Build history of the part. All positions in model axes, mm. Face numbers are marked on the shaded views. Coordinates: 2 decimals unless noted, no trailing zeros. Loops run counter-clockwise (first coordinate to the right, second up) from the corner with the lowest first, then second, coordinate; pieces in that order, holes last. Notation, with made-up numbers: M 25,-29.5 L 61,-29.5 A20 cw 61,-16.5 Z; hole C -11.5,35 d5. An arc over 180 degrees is marked long. Write each question's results on one line, items separated by ' | '. Start each with the question number.
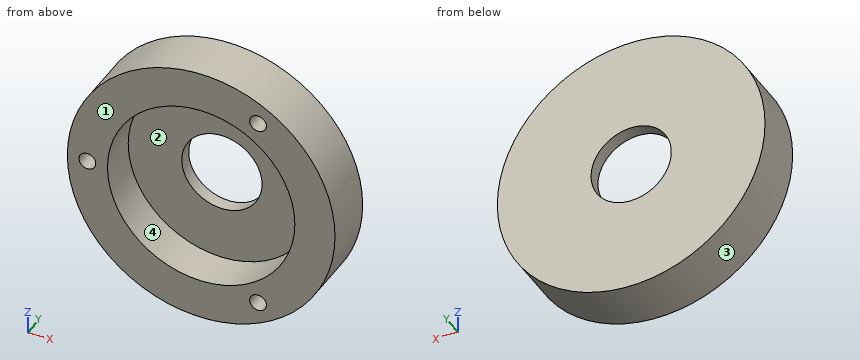
from build123d import *

# Parameters (mm, degrees)
SKETCH1_R                 = 20
BOSS_EXTRUDE1_DEPTH       = 8
SKETCH2_R                 = 14
CUT_EXTRUDE1_DEPTH        = 6
CUT_EXTRUDE4_REACH        = 10
SKETCH3_R                 = 6
M3X0_5_TAPPED_HOLE1_D     = 2.5
M3X0_5_TAPPED_HOLE1_DEPTH = 4
M3X0_5_TAPPED_HOLE1_TIP   = 0.751075774


with BuildPart() as part:
    # Sketch1 → Boss-Extrude1 (new body)
    with BuildSketch(Plane(origin=(0, 3, 0), x_dir=(1, 0, 0), z_dir=(0, 1, 0))):
        with Locations((-34.143225555, -5.12970783)):
            Circle(SKETCH1_R)
    extrude(amount=BOSS_EXTRUDE1_DEPTH)

    # Sketch2 → Cut-Extrude1 (cut)
    with BuildSketch(Plane.XZ.offset(-3)):
        with Locations((-34.143225555, 5.12970783)):
            Circle(SKETCH2_R)
    extrude(amount=-CUT_EXTRUDE1_DEPTH, mode=Mode.SUBTRACT)

    # Sketch3 → Cut-Extrude4 (cut, up to next)
    with BuildSketch(Plane(origin=(0, 11, 0), x_dir=(1, 0, 0), z_dir=(0, 1, 0)), mode=Mode.PRIVATE) as cut_extrude4_sk1:
        with Locations((-34.143225555, -5.12970783)):
            Circle(SKETCH3_R)
    cut_extrude4_tool1 = extrude(cut_extrude4_sk1.sketch, amount=-CUT_EXTRUDE4_REACH, mode=Mode.PRIVATE) & part.part
    add(cut_extrude4_tool1.solids().sort_by_distance((-34.143226, 11, 5.129708))[0], mode=Mode.SUBTRACT)

    # M3x0.5 Tapped Hole1
    with Locations(Plane.XZ.offset(-3)):
        with Locations((-25.643225555, 19.852139695), (-51.143225555, 5.12970783), (-25.643225555, -9.592724034)):
            Hole(M3X0_5_TAPPED_HOLE1_D / 2, depth=M3X0_5_TAPPED_HOLE1_DEPTH)
            with Locations((0, 0, -(M3X0_5_TAPPED_HOLE1_DEPTH + M3X0_5_TAPPED_HOLE1_TIP / 2))):  # 118° drill point
                Cone(0, M3X0_5_TAPPED_HOLE1_D / 2, M3X0_5_TAPPED_HOLE1_TIP, mode=Mode.SUBTRACT)


solid = part.part
1. Mould opens along Z. For the marked faces 1, 2, 3 and 4 say: +Z half, -Z half, draft (parallel to the pull), parting line (faces both ways), or undercut.
2. Band-saw the part on B-B, the plane x = -37. List the corners of the cut face in (y, z).
3. Band-saw the part on D-D, the plane x = -42. List the corners of the cut face in (y, z), plus the area to 3 significant figures.
4. Pin check, flat tips, straight feed: pin 1 (4 mm diameter, centred on x = -38, y = 5, fed in from +Z); pin 2 (7 mm diameter, centred on x = -34.14, z = 5.13, fed in from -Y); pin 3 (8.5 mm diameter, centred on x = -29.5, z = 9, fed in from -Y); pin 4 (3 mm diameter, centred on x = -34.5, y = 7.5, fed in from -Z). Stop position of each tip, or through.
5. Band-saw the part on C-C, the plane y = 10.5. List the corners of the cut face in (x, z).
6. Band-saw the part on A-A, the plane z = 10. List the corners of the cut face in (x, y).
7. Wall check: line 1 along X through (y, z) = (10.25, 8.5); line 2 along Y through (x, z) = (-35, -4); line 3 along X through (y, z) = (4.5, 11.5). Give the ranges that are in metal, low to high.
Checked values:
1) face 1: draft | face 2: undercut | face 3: parting line | face 4: undercut
2) outline: M 3,-14.67 L 11,-14.67 L 11,-0.15 L 9,-0.15 L 9,-8.58 L 3,-8.58 Z; M 3,18.84 L 9,18.84 L 9,10.41 L 11,10.41 L 11,24.92 L 3,24.92 Z
3) outline: M 3,-13.26 L 11,-13.26 L 11,23.52 L 3,23.52 L 3,16.72 L 9,16.72 L 9,-6.46 L 3,-6.46 Z | area: 155 mm²
4) pin 1: z = 25.04 | pin 2: through | pin 3: y = 9 | pin 4: z = -14.87
5) outline: C -34.14,5.13 d40; hole C -34.14,5.13 d12
6) outline: M -53.54,3 L -47.27,3 L -47.27,9 L -37.65,9 L -37.65,11 L -53.54,11 Z; M -30.64,9 L -21.02,9 L -21.02,3 L -14.75,3 L -14.75,11 L -30.64,11 Z
7) line 1: -53.86 to -39.11, -29.18 to -14.43 | line 2: 9 to 11 | line 3: -53.1 to -46.61, -21.68 to -15.18
